Build history of the part. All positions in model axes, mm. Round coordinates to 2 decimals unless told otherwise and drop trailing zeros. Order: outer loops, then holes, each group sorted by start corner. A loop starts at its lowest first (then second) coordinate and runs counter-clockwise, first axis right, second up. Notation, with made-up numbers: M -39.75,-28 L -8.75,-28 A18 cw -8.75,-22 Z; hole C 58,28 d3. An arc over 180 degrees is marked long. One line per question, with ' | ' between items. Start each with the question number.
from build123d import *

# Parameters (mm, degrees)
SKETCH1_W           = 1117.6
SKETCH1_H           = 501.65
BOSS_EXTRUDE1_DEPTH = 11.90625
SKETCH3_R           = 15.875
CUT_EXTRUDE1_DEPTH  = 613.627439325
CHAMFER1_SIZE       = 139.7
CHAMFER1_SIZE2      = 241.967497817


with BuildPart() as part:
    # Sketch1 → Boss-Extrude1 (new body)
    with BuildSketch(Plane(origin=(0, 0, 0), x_dir=(0, 0, -1), z_dir=(1, 0, 0))):
        Rectangle(SKETCH1_W, SKETCH1_H)
    extrude(amount=BOSS_EXTRUDE1_DEPTH)

    # Sketch3 → Cut-Extrude1 (cut, through all)
    with BuildSketch(Plane(origin=(11.90625, 0, 0), x_dir=(0, 0, -1), z_dir=(1, 0, 0))):
        with Locations((-508, 212.725)):
            Circle(SKETCH3_R)
        with Locations((508, 212.725)):
            Circle(SKETCH3_R)
    extrude(amount=-CUT_EXTRUDE1_DEPTH, mode=Mode.SUBTRACT)

    # Chamfer1
    chamfer1_edges = [part.edges().sort_by_distance(p)[0] for p in [
        (5.953125, -250.825, -558.8),
        (5.953125, -250.825, 558.8),
    ]]
    chamfer1_side = [part.faces().sort_by_distance(p)[0] for p in [
        (5.953125, -250.825, 0),
    ]]
    chamfer(chamfer1_edges, length=CHAMFER1_SIZE, length2=CHAMFER1_SIZE2, reference=chamfer1_side[0])


solid = part.part
Item 1: Cut at B-B on z = -508. Write the cut outline in (x, y) (3 decimals).
Item 2: Cut at D-D on z = 475. Write the cut outline in (x, y) (3 decimals), then the cut area to 3 significant figures.
Item 3: Wall check: line 1 along Y through (x, z) = (3.25, 508) (3 decimals); line 2 along Z through (x, y) = (5, -169); line 3 along Y through (x, z) = (5.5, -430) (3 decimals). Give the ranges that are in metal, low to high. Write a range as [from, to].
Item 4: Cut at A-A on x = 6.25. Count the separate pieces of the cut face and the enclosed holes in it, then the cut area to 3 significant figures.
Item 5: Cut at C-C on y = -98. Write the cut outline in (x, z), then the cut area to 3 significant figures.
Item 6: Two-plate mould, pull along Z, no slides. Class faces 1 (the face through (6.036, 197.228, -504.559)), 2 (the face through (5.87, -128.147, -489.928)), 3 (the face through (0, 4, 8)): +Z half, -Z half, draft (parallel to the pull), parting line (faces both ways), or undercut.
Results found:
1) outline: M 0,-96.846 L 11.906,-96.846 L 11.906,196.85 L 0,196.85 Z; M 0,228.6 L 11.906,228.6 L 11.906,250.825 L 0,250.825 Z
2) outline: M 0,-154.003 L 11.906,-154.003 L 11.906,250.825 L 0,250.825 Z | area: 4,820 mm^2
3) line 1: y = [-96.846, 196.85], [228.6, 250.825] | line 2: z = [-466.34, 466.34] | line 3: y = [-231.946, 250.825]
4) separate pieces: 1 | enclosed holes: 2 | area: 525,000 mm^2
5) outline: M 0,-507.33 L 11.91,-507.33 L 11.91,507.33 L 0,507.33 Z | area: 12,100 mm^2
6) face 1: undercut | face 2: -Z half | face 3: draft
